Source: CAD feature listing. Evaluate the final solid. Frame: model axes, mm. Face numbers are marked on the shaded views. Round coordinates to 2 decimals unless told otherwise and drop trailing zeros. Loops run counter-clockwise (first coordinate to the right, second up) from the corner with the lowest first, then second, coordinate; pieces in that order, holes last.
(1) Section C-C, the plane z = 1. Return the cut outline in (x, y), plus the area to 3 significant figures.
(2) First-contact query: pin 1 Ø6 at (x, y) = (-99.66, -13.97) entering from +Z; pin 2 Ø1.1 at (x, z) = (-46, 7) entering from +Y. Flat tips, straight axial feed; report the tip coordinate or a pass-through.
(3) Mould query, pull axis Y, two halves, no side actions, for the marked faces 1, 2 and 3. Classes: pulls with the +Y half, pulls with the -Y half, needs draft (parallel to the pull), parting line crosses it, or undercut.
(4) Section B-B, the plane x = -82. Return the cut outline in (y, z), plus the area to 3 significant figures.
(5) Material intervals for probe 1 along Y at (x, z) = (-57.5, 12.5); probe 2 along Y at (x, z) = (-82, 7.75); probe 3 along Z at (x, y) = (-37, -86), sorted ascending.
(6) Section A-A, the plane y = -45.5. Return the cut outline in (x, z), plus the area to 3 significant figures.
(7) Section D-D, the plane z = 6.75. Return the cut outline in (x, y).
```python
from build123d import *

# Parameters (mm, degrees)
F0_R     = 2.25
F0_R_2   = 38.5
F1_DEPTH = 15
F2_W     = 67
F2_H     = 3.7
F3_DEPTH = 78


with BuildPart() as f1:
    # F0 (on Top) → F1 (new body)
    with BuildSketch(Plane.XY):
        with BuildLine():
            ThreePointArc((-22.661046, -11.973848), (-23.539726, -9.852527), (-25.661046, -8.973848))
            Line((-25.661046, -8.973848), (-101.661046, -8.973848))
            ThreePointArc((-101.661046, -8.973848), (-103.782367, -9.852527), (-104.661046, -11.973848))
            Line((-104.661046, -11.973848), (-104.661046, -87.973848))
            ThreePointArc((-104.661046, -87.973848), (-103.782367, -90.095168), (-101.661046, -90.973848))
            Line((-101.661046, -90.973848), (-25.661046, -90.973848))
            ThreePointArc((-25.661046, -90.973848), (-23.539726, -90.095168), (-22.661046, -87.973848))
            Line((-22.661046, -87.973848), (-22.661046, -11.973848))
        make_face()
        with Locations((-99.261046, -86.573848)):
            Circle(F0_R, mode=Mode.SUBTRACT)
        with Locations((-28.061046, -86.573848)):
            Circle(F0_R, mode=Mode.SUBTRACT)
        with Locations((-63.661046, -49.973848)):
            Circle(F0_R_2, mode=Mode.SUBTRACT)
        with Locations((-99.661046, -13.973848)):
            Circle(F0_R, mode=Mode.SUBTRACT)
        with Locations((-28.061046, -15.373848)):
            Circle(F0_R, mode=Mode.SUBTRACT)
    extrude(amount=F1_DEPTH)

    # F2 (on face) → F3 (cut)
    with BuildSketch(Plane(origin=(0, -8.973848, 0), x_dir=(-1, 0, 0), z_dir=(0, 1, 0))):
        with Locations((63.661046, 7.5)):
            Rectangle(F2_W, F2_H)
    extrude(amount=-F3_DEPTH, mode=Mode.SUBTRACT)


solid = f1.part
```
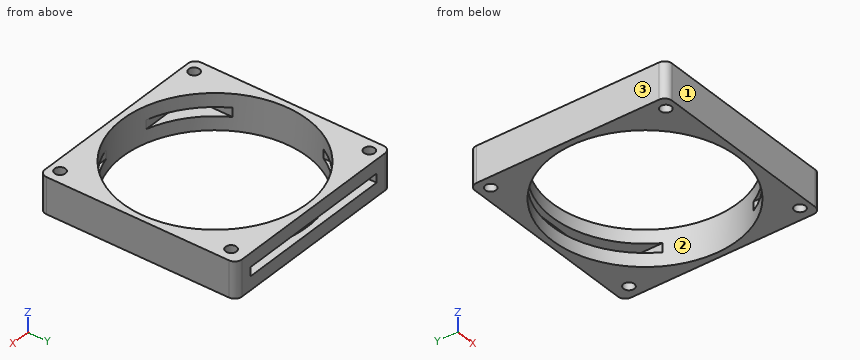
Output values:
1. outline: (-104.66, -87.97) arc R3 ccw to (-101.66, -90.97) - (-25.66, -90.97) arc R3 ccw to (-22.66, -87.97) - (-22.66, -11.97) arc R3 ccw to (-25.66, -8.97) - (-101.66, -8.97) arc R3 ccw to (-104.66, -11.97) - close; hole circle Ø77 at (-63.66, -49.97); hole circle Ø4.5 at (-99.66, -13.97); hole circle Ø4.5 at (-99.26, -86.57); hole circle Ø4.5 at (-28.06, -86.57); hole circle Ø4.5 at (-28.06, -15.37)
1. area: 2,000 mm2
2. pin 1: stops at z = 15
2. pin 2: stops at y = -86.97
3. face 1: pulls with the -Y half
3. face 2: undercut
3. face 3: needs draft
4. outline: (-90.97, 0) - (-83.83, 0) - (-83.83, 5.65) - (-86.97, 5.65) - (-86.97, 9.35) - (-83.83, 9.35) - (-83.83, 15) - (-90.97, 15) - close; (-16.12, 0) - (-8.97, 0) - (-8.97, 5.65) - (-16.12, 5.65) - close; (-16.12, 9.35) - (-8.97, 9.35) - (-8.97, 15) - (-16.12, 15) - close
4. area: 176 mm2
5. probe 1: y = -90.97 to -87.98, -11.97 to -8.97
5. probe 2: y = -90.97 to -86.97
5. probe 3: z = 0 to 5.65, 9.35 to 15
6. outline: (-104.66, 0) - (-101.9, 0) - (-101.9, 15) - (-104.66, 15) - close; (-25.42, 0) - (-22.66, 0) - (-22.66, 15) - (-25.42, 15) - close
6. area: 82.8 mm2
7. outline: (-104.66, -87.97) arc R3 ccw to (-101.66, -90.97) - (-25.66, -90.97) arc R3 ccw to (-22.66, -87.97) - (-22.66, -11.97) arc R3 ccw to (-25.66, -8.97) - (-30.16, -8.97) - (-30.16, -14.57) arc R2.25 cw (long way) to (-30.16, -16.18) - (-30.16, -31) arc R38.5 cw to (-30.16, -68.95) - (-30.16, -85.77) arc R2.25 cw (long way) to (-30.28, -86.97) - (-53.02, -86.97) arc R38.5 cw to (-74.3, -86.97) - (-97.05, -86.97) arc R2.25 cw (long way) to (-97.16, -85.77) - (-97.16, -68.95) arc R38.5 cw to (-97.16, -31) - (-97.16, -8.97) - (-101.66, -8.97) arc R3 ccw to (-104.66, -11.97) - close; hole circle Ø4.5 at (-99.66, -13.97)
